Read the model definition and answer for the solid it produces. Units are mm, in the model's axes. A direction names the side the tool comes from. Give positions to 0.01 mm unless a question says otherwise; leave off trailing zeros. Order: outer loops, then holes, each group sorted by start corner. A loop starts at its lowest first (then second) coordinate and runs counter-clockwise, first axis right, second up.
```python
from build123d import *

# Parameters (mm, degrees)
F0_W     = 558.8
F0_H     = 1524
F1_DEPTH = 76.2
F2_R     = 50.8
F3_DEPTH = 685.8
F5_DEPTH = 76.2
F6_R     = 127


with BuildPart() as f1:
    # F0 (on Top) → F1 (new body)
    with BuildSketch(Plane.XY):
        Rectangle(F0_W, F0_H)
    extrude(amount=F1_DEPTH)

    # F2 (on face) → F3 (join)
    with BuildSketch(Plane(origin=(0, 0, 0), x_dir=(1, 0, 0), z_dir=(0, 0, -1))):
        with Locations((-203.2, -685.8)):
            Circle(F2_R)
        with Locations((203.2, -685.8)):
            Circle(F2_R)
        with Locations((203.231033, 685.8)):
            Circle(F2_R)
        with Locations((-203.2, 685.8)):
            Circle(F2_R)
    extrude(amount=F3_DEPTH)

    # F4 (on face) → F5 (join)
    with BuildSketch(Plane.XY.offset(76.2)):
        Polygon((-279.4, 635), (-279.4, 762), (-533.4, 762), (-533.4, -762), (-279.4, -762), (-279.4, -635), (-304.8, -635), (-304.8, 635), align=None)
        Polygon((533.4, 762), (279.4, 762), (279.4, 635), (304.8, 635), (304.8, -635), (279.4, -635), (279.4, -762), (533.4, -762), align=None)
    extrude(amount=-F5_DEPTH)

    # F6
    f6_edges = [f1.edges().sort_by_distance(p)[0] for p in [
        (-533.4, -762, 38.1),
        (533.4, -762, 38.1),
        (533.4, 762, 38.1),
        (-533.4, 762, 38.1),
    ]]
    fillet(f6_edges, radius=F6_R)


solid = f1.part
```
1) The part is cut by section B-B on z = -72.5. Determine the outline of the cut face in (x, y), and give its area (3 significant figures).
Final values:
outline: circle Ø101.6 at (-203.2, -685.8); circle Ø101.6 at (-203.2, 685.8); circle Ø101.6 at (203.2, 685.8); circle Ø101.6 at (203.23, -685.8)
area: 32,400 mm2
2) A tool of negligible diameter and unlimited length cuts with its end or side. For faces 5 (the face through (-7, 11, 0)), 6 (the face through (-7, 11, 76.2)), 7 (the face through (304.8, 9, 39)), from which of +Z, -Z, +X, -X, +Y, -Y can it reach the whole face along a straight path? Write none if from no direction.
Final values:
face 5: -Z
face 6: +Z, +X, -X, +Y, -Y
face 7: +Z, -Z
3) The part is cut by section C-C on x = 203.2. Determine the outline of the cut face in (y, z).
Final values:
outline: (-762, 0) - (-736.6, 0) - (-736.6, -685.8) - (-635, -685.8) - (-635, 0) - (635, 0) - (635, -685.8) - (736.6, -685.8) - (736.6, 0) - (762, 0) - (762, 76.2) - (-762, 76.2) - close
4) For a pull along X with two mould halves and no side action, classify faces 1 (the face through (-495.21, 725.785, 37.567)), 2 (the face through (495.21, 725.785, 37.567)), 3 (the face through (-6, -762, 39)), 4 (the face through (-279.4, -9, 38)) as released by +X, released by -X, zero draft, split by the parting line, or undercut.
Final values:
face 1: released by -X
face 2: released by +X
face 3: zero draft
face 4: undercut
5) The part is cut by section A-A on y = 448. Determine the outline of the cut face in (x, z).
Final values:
outline: (-533.4, 0) - (-304.8, 0) - (-304.8, 76.2) - (-533.4, 76.2) - close; (-279.4, 0) - (279.4, 0) - (279.4, 76.2) - (-279.4, 76.2) - close; (304.8, 0) - (533.4, 0) - (533.4, 76.2) - (304.8, 76.2) - close
6) Consider L1, parallel to X at y = 26.5, z = 27; L2, parallel to Z at x = 365, y = -584; L3, parallel to X at y = -682, z = -343.5. Determine where each line is inside the solid, lowest interval first.
Final values:
L1: x = -533.4 to -304.8, -279.4 to 279.4, 304.8 to 533.4
L2: z = 0 to 76.2
L3: x = -253.86 to -152.54, 152.57 to 253.89
